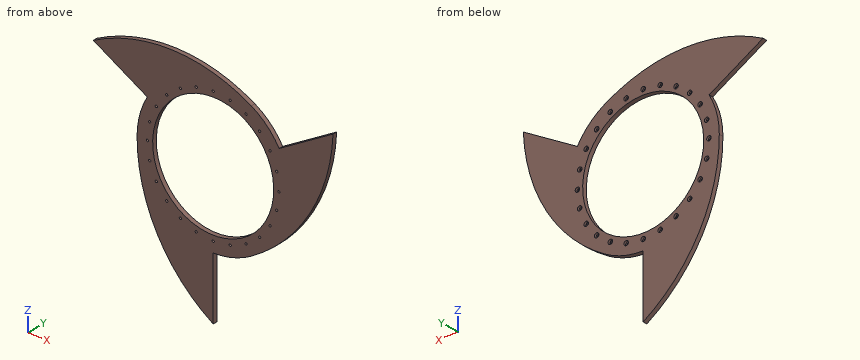
```python
from build123d import *

# Parameters (mm, degrees)
SKETCH1_R                      = 87.5
BOSS_EXTRUDE1_DEPTH            = 6.35
CBORE_FOR_M3_SHCS1_AT_2_COUNT  = 2
CBORE_FOR_M3_SHCS1_AT_2_PITCH  = 24.799976522
CBORE_FOR_M3_SHCS1_AT_3_COUNT  = 2
CBORE_FOR_M3_SHCS1_AT_3_PITCH  = 49.175618569
CBORE_FOR_M3_SHCS1_AT_4_COUNT  = 2
CBORE_FOR_M3_SHCS1_AT_4_PITCH  = 72.709852149
CBORE_FOR_M3_SHCS1_AT_5_COUNT  = 2
CBORE_FOR_M3_SHCS1_AT_5_PITCH  = 95
CBORE_FOR_M3_SHCS1_AT_6_COUNT  = 2
CBORE_FOR_M3_SHCS1_AT_6_PITCH  = 115.664671512
CBORE_FOR_M3_SHCS1_AT_7_COUNT  = 2
CBORE_FOR_M3_SHCS1_AT_7_PITCH  = 134.350288425
CBORE_FOR_M3_SHCS1_AT_8_COUNT  = 2
CBORE_FOR_M3_SHCS1_AT_8_PITCH  = 150.737134655
CBORE_FOR_M3_SHCS1_AT_9_COUNT  = 2
CBORE_FOR_M3_SHCS1_AT_9_PITCH  = 164.544826719
CBORE_FOR_M3_SHCS1_AT_10_COUNT = 2
CBORE_FOR_M3_SHCS1_AT_10_PITCH = 175.537111177
CBORE_FOR_M3_SHCS1_AT_11_COUNT = 2
CBORE_FOR_M3_SHCS1_AT_11_PITCH = 183.525906995
CBORE_FOR_M3_SHCS1_AT_12_COUNT = 2
CBORE_FOR_M3_SHCS1_AT_12_PITCH = 188.374523661
CBORE_FOR_M3_SHCS1_AT_13_COUNT = 2
CBORE_FOR_M3_SHCS1_AT_13_PITCH = 190
CBORE_FOR_M3_SHCS1_AT_14_COUNT = 2
CBORE_FOR_M3_SHCS1_AT_14_PITCH = 188.374523661
CBORE_FOR_M3_SHCS1_AT_15_COUNT = 2
CBORE_FOR_M3_SHCS1_AT_15_PITCH = 183.525906995
CBORE_FOR_M3_SHCS1_AT_16_COUNT = 2
CBORE_FOR_M3_SHCS1_AT_16_PITCH = 175.537111177
CBORE_FOR_M3_SHCS1_AT_17_COUNT = 2
CBORE_FOR_M3_SHCS1_AT_17_PITCH = 164.544826719
CBORE_FOR_M3_SHCS1_AT_18_COUNT = 2
CBORE_FOR_M3_SHCS1_AT_18_PITCH = 150.737134655
CBORE_FOR_M3_SHCS1_AT_19_COUNT = 2
CBORE_FOR_M3_SHCS1_AT_19_PITCH = 134.350288425
CBORE_FOR_M3_SHCS1_AT_20_COUNT = 2
CBORE_FOR_M3_SHCS1_AT_20_PITCH = 115.664671512
CBORE_FOR_M3_SHCS1_AT_21_COUNT = 2
CBORE_FOR_M3_SHCS1_AT_21_PITCH = 95
CBORE_FOR_M3_SHCS1_AT_22_COUNT = 2
CBORE_FOR_M3_SHCS1_AT_22_PITCH = 72.709852149
CBORE_FOR_M3_SHCS1_AT_23_COUNT = 2
CBORE_FOR_M3_SHCS1_AT_23_PITCH = 49.175618569
CBORE_FOR_M3_SHCS1_AT_24_COUNT = 2
CBORE_FOR_M3_SHCS1_AT_24_PITCH = 24.799976522
CBORE_FOR_M3_SHCS1_AT_25_COUNT = 2
CBORE_FOR_M3_SHCS1_AT_25_PITCH = 95


with BuildPart() as part:
    # Sketch1 → Boss-Extrude1 (new body)
    with BuildSketch(Plane(origin=(0, 0, 0), x_dir=(1, 0, 0), z_dir=(0, 1, 0))):
        with BuildLine():
            Line((0, 200), (0, 110))
            ThreePointArc((0, 110), (28.470094961, 106.251840892), (55, 95.262794416))
            ThreePointArc((55, 95.262794416), (139.179825281, 12.812284565), (173.205080757, -100))
            Line((173.205080757, -100), (95.262794416, -55))
            ThreePointArc((95.262794416, -55), (77.781745931, -77.781745931), (55, -95.262794416))
            ThreePointArc((55, -95.262794416), (-58.494148726, -126.939406671), (-173.205080757, -100))
            Line((-173.205080757, -100), (-95.262794416, -55))
            ThreePointArc((-95.262794416, -55), (-106.251840892, -28.470094961), (-110, 0))
            ThreePointArc((-110, 0), (-80.685676555, 114.127122105), (0, 200))
        make_face()
        with Locations(Location((0, 0, 0), (0, 0, 270))):
            Circle(SKETCH1_R, mode=Mode.SUBTRACT)
    extrude(amount=BOSS_EXTRUDE1_DEPTH)

    # Sketch3 → CBORE for M3 SHCS1 (revolve, cut)
    with BuildSketch(Plane(origin=(95, 6.35, 0), x_dir=(0, 0, 1), z_dir=(1, 0, 0))):
        Polygon((0, 0), (0, 6.35), (1.6, 6.35), (1.6, 3), (3.25, 3), (3.25, 0.025), (3.275, 0), align=None)
    cbore_for_m3_shcs1 = revolve(axis=Axis((95, 12.7, 0), (0, -1, 0)), mode=Mode.SUBTRACT)

    # CBORE for M3 SHCS1 at 2: CBORE for M3 SHCS1 ×2
    with Locations(*[Vector(-0.1305261922200521, 0, 0.9914448613738104) * (i * CBORE_FOR_M3_SHCS1_AT_2_PITCH) for i in range(1, CBORE_FOR_M3_SHCS1_AT_2_COUNT)]):
        add(cbore_for_m3_shcs1, mode=Mode.SUBTRACT)

    # CBORE for M3 SHCS1 at 3: CBORE for M3 SHCS1 ×2
    with Locations(*[Vector(-0.2588190451025218, 0, 0.965925826289068) * (i * CBORE_FOR_M3_SHCS1_AT_3_PITCH) for i in range(1, CBORE_FOR_M3_SHCS1_AT_3_COUNT)]):
        add(cbore_for_m3_shcs1, mode=Mode.SUBTRACT)

    # CBORE for M3 SHCS1 at 4: CBORE for M3 SHCS1 ×2
    with Locations(*[Vector(-0.38268343236509056, 0, 0.9238795325112865) * (i * CBORE_FOR_M3_SHCS1_AT_4_PITCH) for i in range(1, CBORE_FOR_M3_SHCS1_AT_4_COUNT)]):
        add(cbore_for_m3_shcs1, mode=Mode.SUBTRACT)

    # CBORE for M3 SHCS1 at 5: CBORE for M3 SHCS1 ×2
    with Locations(*[Vector(-0.5000000000000009, 0, 0.8660254037844382) * (i * CBORE_FOR_M3_SHCS1_AT_5_PITCH) for i in range(1, CBORE_FOR_M3_SHCS1_AT_5_COUNT)]):
        add(cbore_for_m3_shcs1, mode=Mode.SUBTRACT)

    # CBORE for M3 SHCS1 at 6: CBORE for M3 SHCS1 ×2
    with Locations(*[Vector(-0.6087614290087218, 0, 0.7933533402912344) * (i * CBORE_FOR_M3_SHCS1_AT_6_PITCH) for i in range(1, CBORE_FOR_M3_SHCS1_AT_6_COUNT)]):
        add(cbore_for_m3_shcs1, mode=Mode.SUBTRACT)

    # CBORE for M3 SHCS1 at 7: CBORE for M3 SHCS1 ×2
    with Locations(*[Vector(-0.7071067811865487, 0, 0.7071067811865464) * (i * CBORE_FOR_M3_SHCS1_AT_7_PITCH) for i in range(1, CBORE_FOR_M3_SHCS1_AT_7_COUNT)]):
        add(cbore_for_m3_shcs1, mode=Mode.SUBTRACT)

    # CBORE for M3 SHCS1 at 8: CBORE for M3 SHCS1 ×2
    with Locations(*[Vector(-0.7933533402912363, 0, 0.6087614290087191) * (i * CBORE_FOR_M3_SHCS1_AT_8_PITCH) for i in range(1, CBORE_FOR_M3_SHCS1_AT_8_COUNT)]):
        add(cbore_for_m3_shcs1, mode=Mode.SUBTRACT)

    # CBORE for M3 SHCS1 at 9: CBORE for M3 SHCS1 ×2
    with Locations(*[Vector(-0.8660254037844398, 0, 0.499999999999998) * (i * CBORE_FOR_M3_SHCS1_AT_9_PITCH) for i in range(1, CBORE_FOR_M3_SHCS1_AT_9_COUNT)]):
        add(cbore_for_m3_shcs1, mode=Mode.SUBTRACT)

    # CBORE for M3 SHCS1 at 10: CBORE for M3 SHCS1 ×2
    with Locations(*[Vector(-0.9238795325112878, 0, 0.3826834323650874) * (i * CBORE_FOR_M3_SHCS1_AT_10_PITCH) for i in range(1, CBORE_FOR_M3_SHCS1_AT_10_COUNT)]):
        add(cbore_for_m3_shcs1, mode=Mode.SUBTRACT)

    # CBORE for M3 SHCS1 at 11: CBORE for M3 SHCS1 ×2
    with Locations(*[Vector(-0.9659258262890691, 0, 0.25881904510251796) * (i * CBORE_FOR_M3_SHCS1_AT_11_PITCH) for i in range(1, CBORE_FOR_M3_SHCS1_AT_11_COUNT)]):
        add(cbore_for_m3_shcs1, mode=Mode.SUBTRACT)

    # CBORE for M3 SHCS1 at 12: CBORE for M3 SHCS1 ×2
    with Locations(*[Vector(-0.9914448613738108, 0, 0.13052619222004846) * (i * CBORE_FOR_M3_SHCS1_AT_12_PITCH) for i in range(1, CBORE_FOR_M3_SHCS1_AT_12_COUNT)]):
        add(cbore_for_m3_shcs1, mode=Mode.SUBTRACT)

    # CBORE for M3 SHCS1 at 13: CBORE for M3 SHCS1 ×2
    with Locations(*[(-i * CBORE_FOR_M3_SHCS1_AT_13_PITCH, 0, 0) for i in range(1, CBORE_FOR_M3_SHCS1_AT_13_COUNT)]):
        add(cbore_for_m3_shcs1, mode=Mode.SUBTRACT)

    # CBORE for M3 SHCS1 at 14: CBORE for M3 SHCS1 ×2
    with Locations(*[Vector(-0.9914448613738099, 0, -0.13052619222005532) * (i * CBORE_FOR_M3_SHCS1_AT_14_PITCH) for i in range(1, CBORE_FOR_M3_SHCS1_AT_14_COUNT)]):
        add(cbore_for_m3_shcs1, mode=Mode.SUBTRACT)

    # CBORE for M3 SHCS1 at 15: CBORE for M3 SHCS1 ×2
    with Locations(*[Vector(-0.9659258262890673, 0, -0.25881904510252474) * (i * CBORE_FOR_M3_SHCS1_AT_15_PITCH) for i in range(1, CBORE_FOR_M3_SHCS1_AT_15_COUNT)]):
        add(cbore_for_m3_shcs1, mode=Mode.SUBTRACT)

    # CBORE for M3 SHCS1 at 16: CBORE for M3 SHCS1 ×2
    with Locations(*[Vector(-0.9238795325112852, 0, -0.38268343236509383) * (i * CBORE_FOR_M3_SHCS1_AT_16_PITCH) for i in range(1, CBORE_FOR_M3_SHCS1_AT_16_COUNT)]):
        add(cbore_for_m3_shcs1, mode=Mode.SUBTRACT)

    # CBORE for M3 SHCS1 at 17: CBORE for M3 SHCS1 ×2
    with Locations(*[Vector(-0.8660254037844364, 0, -0.5000000000000039) * (i * CBORE_FOR_M3_SHCS1_AT_17_PITCH) for i in range(1, CBORE_FOR_M3_SHCS1_AT_17_COUNT)]):
        add(cbore_for_m3_shcs1, mode=Mode.SUBTRACT)

    # CBORE for M3 SHCS1 at 18: CBORE for M3 SHCS1 ×2
    with Locations(*[Vector(-0.7933533402912322, 0, -0.6087614290087247) * (i * CBORE_FOR_M3_SHCS1_AT_18_PITCH) for i in range(1, CBORE_FOR_M3_SHCS1_AT_18_COUNT)]):
        add(cbore_for_m3_shcs1, mode=Mode.SUBTRACT)

    # CBORE for M3 SHCS1 at 19: CBORE for M3 SHCS1 ×2
    with Locations(*[Vector(-0.7071067811865438, 0, -0.7071067811865513) * (i * CBORE_FOR_M3_SHCS1_AT_19_PITCH) for i in range(1, CBORE_FOR_M3_SHCS1_AT_19_COUNT)]):
        add(cbore_for_m3_shcs1, mode=Mode.SUBTRACT)

    # CBORE for M3 SHCS1 at 20: CBORE for M3 SHCS1 ×2
    with Locations(*[Vector(-0.6087614290087162, 0, -0.7933533402912386) * (i * CBORE_FOR_M3_SHCS1_AT_20_PITCH) for i in range(1, CBORE_FOR_M3_SHCS1_AT_20_COUNT)]):
        add(cbore_for_m3_shcs1, mode=Mode.SUBTRACT)

    # CBORE for M3 SHCS1 at 21: CBORE for M3 SHCS1 ×2
    with Locations(*[Vector(-0.4999999999999949, 0, -0.8660254037844416) * (i * CBORE_FOR_M3_SHCS1_AT_21_PITCH) for i in range(1, CBORE_FOR_M3_SHCS1_AT_21_COUNT)]):
        add(cbore_for_m3_shcs1, mode=Mode.SUBTRACT)

    # CBORE for M3 SHCS1 at 22: CBORE for M3 SHCS1 ×2
    with Locations(*[Vector(-0.3826834323650841, 0, -0.9238795325112891) * (i * CBORE_FOR_M3_SHCS1_AT_22_PITCH) for i in range(1, CBORE_FOR_M3_SHCS1_AT_22_COUNT)]):
        add(cbore_for_m3_shcs1, mode=Mode.SUBTRACT)

    # CBORE for M3 SHCS1 at 23: CBORE for M3 SHCS1 ×2
    with Locations(*[Vector(-0.25881904510251497, 0, -0.9659258262890699) * (i * CBORE_FOR_M3_SHCS1_AT_23_PITCH) for i in range(1, CBORE_FOR_M3_SHCS1_AT_23_COUNT)]):
        add(cbore_for_m3_shcs1, mode=Mode.SUBTRACT)

    # CBORE for M3 SHCS1 at 24: CBORE for M3 SHCS1 ×2
    with Locations(*[Vector(-0.1305261922200453, 0, -0.9914448613738113) * (i * CBORE_FOR_M3_SHCS1_AT_24_PITCH) for i in range(1, CBORE_FOR_M3_SHCS1_AT_24_COUNT)]):
        add(cbore_for_m3_shcs1, mode=Mode.SUBTRACT)

    # CBORE for M3 SHCS1 at 25: CBORE for M3 SHCS1 ×2
    with Locations(*[(-i * CBORE_FOR_M3_SHCS1_AT_25_PITCH, 0, 0) for i in range(1, CBORE_FOR_M3_SHCS1_AT_25_COUNT)]):
        add(cbore_for_m3_shcs1, mode=Mode.SUBTRACT)


solid = part.part
```
Build history of the part. All positions in model axes, mm. Give positions to 0.01 mm unless a question says otherwise; leave off trailing zeros. Order: outer loops, then holes, each group sorted by start corner. A loop starts at its lowest first (then second) coordinate and runs counter-clockwise, first axis right, second up. Notation, with made-up numbers: M -3.75,48.5 L 19.25,48.5 A10 cw 19.25,64.5 Z; hole C 38,-37 d11. An arc over 180 degrees is marked long. Write item = value, one per line. Start each with the question number.
(1) Slice it at A-A on y = 1.75. State how many separate pieces and enclosed holes the cut face has, plus the area to 3 significant figures.
(2) Probe L1, parallel to Z at x = 65.5, y = 5.25; L2, parallel to X at y = 1.45, z = 0; L3, parallel to X at y = 5.5, z = -47.5. List the from-to ranges inside material, lowest first. Write a range as [from, to].
(3) Slice it at B-B on z = -153.5. Write the cut outline in (x, y).
(4) Pin check, flat tips, straight feed: pin 1 Ø1.5 at (y, z) = (3, -142) entering from +X; pin 2 Ø1.9 at (x, z) = (-82.27, 47.5) entering from -Y; pin 3 Ø2 at (y, z) = (5, -55.5) entering from +X; pin 4 Ø2 at (x, z) = (-47, 81) entering from +Y. Stop position of each tip, or through.
(5) Slice it at C-C on x = -124.5. Write the cut outline in (y, z), plus the area to 3 significant figures.
Responses:
q1.separate_pieces = 1
q1.enclosed_holes = 25
q1.area = 31,800 mm2
q2.L1 = [-88.83, -69.96], [-64.39, -58.02], [58.02, 64.39], [69.96, 88.37]
q2.L2 = [-110, -96.6], [-93.4, -87.5], [87.5, 93.4], [96.6, 146.4]
q2.L3 = [-105.19, -85.52], [-79.02, -73.48], [73.48, 79.02], [85.52, 113.6]
q3.outline = M -53.52,0 L 0,0 L 0,6.35 L -53.52,6.35 Z
q4.pin_1 = 0
q4.pin_2 = through
q4.pin_3 = 107.12
q4.pin_4 = 3.35
q5.outline = M 0,71.88 L 6.35,71.88 L 6.35,118.98 L 0,118.98 Z
q5.area = 299 mm2
